from build123d import *

# Parameters (mm, degrees)
SKETCH_1_R          = 1.35
EXTRUDE_1_DEPTH     = 12.5
SKETCH_3_R          = 9
SKETCH_4_R          = 9.9
SKETCH_4_R_2        = 9
EXTRUDE_2_DEPTH     = 1
CUT_EXTRUDE_START   = -2
SKETCH_5_R          = 13.5
SKETCH_5_R_2        = 9.9
CUT_EXTRUDE_1_DEPTH = 2
SKETCH_6_R          = 10.1
CUT_EXTRUDE_2_DEPTH = 3.25
SKETCH_10_R         = 1.35
CUT_EXTRUDE_3_DEPTH = 8
CUT_EXTRUDE_4_REACH = 60.397
SKETCH_11_R         = 1.6
SKETCH_12_R         = 3
CUT_EXTRUDE_5_DEPTH = 4


with BuildPart() as part:
    # 草图1 → 凸台-拉伸1 (new, symmetric)
    with BuildSketch(Plane.XY):
        Polygon((0, 0), (0, 39.5), (-19, 39.5), (-35, 23.5), (-35, -20), (-17, -38), (0, -38), align=None)
        with Locations((-27.980762114, -15)):
            Circle(SKETCH_1_R, mode=Mode.SUBTRACT)
        with Locations((-23.213203436, -21.213203436)):
            Circle(SKETCH_1_R, mode=Mode.SUBTRACT)
        with Locations((-17, -25.980762114)):
            Circle(SKETCH_1_R, mode=Mode.SUBTRACT)
        with Locations((-9.764571353, -28.977774789)):
            Circle(SKETCH_1_R, mode=Mode.SUBTRACT)
        with Locations((-30.070163865, 15.944644586)):
            Circle(SKETCH_1_R, mode=Mode.SUBTRACT)
        with Locations((-26.212865417, 23.354445963)):
            Circle(SKETCH_1_R, mode=Mode.SUBTRACT)
        with Locations((-20.56920351, 29.51342218)):
            Circle(SKETCH_1_R, mode=Mode.SUBTRACT)
    extrude(amount=EXTRUDE_1_DEPTH, both=True)

    # 切除-扫描1: sweep along a path in 草图2
    with BuildLine(Plane.XY) as sweep_1_path:
        Line((0, -18), (-2, -18))
        ThreePointArc((-2, -18), (-14.727922061, -12.727922061), (-20, 0))
        Line((-20, 0), (-20, 5))
        ThreePointArc((-20, 5), (-17.320508076, 15), (-10, 22.320508076))
        ThreePointArc((-10, 22.320508076), (3.381115126, 27.650519119), (17.726426944, 28.94484851))
    # 草图3 → 切除-扫描1 (sweep, cut)
    with BuildSketch(Plane(origin=(0, 0, 0), x_dir=(0, 0, -1), z_dir=(1, 0, 0))):
        with Locations((0, -18)):
            Circle(SKETCH_3_R)
    sweep(path=sweep_1_path.line, mode=Mode.SUBTRACT)

    # 草图4 → 凸台-拉伸2 (add)
    with BuildSketch(Plane(origin=(0, 0, 0), x_dir=(0, 0, -1), z_dir=(1, 0, 0))):
        with Locations(Location((0, -18, 0), (0, 0, 180))):
            Circle(SKETCH_4_R)
        with Locations((0, -18)):
            Circle(SKETCH_4_R_2, mode=Mode.SUBTRACT)
    extrude(amount=EXTRUDE_2_DEPTH)

    # 草图5 → 切除-拉伸1 (cut)
    with BuildSketch(Plane(origin=(0, 0, 0), x_dir=(0, 0, -1), z_dir=(1, 0, 0)).offset(CUT_EXTRUDE_START)):
        with Locations((0, -18)):
            Circle(SKETCH_5_R)
        with Locations((0, -18)):
            Circle(SKETCH_5_R_2, mode=Mode.SUBTRACT)
    extrude(amount=CUT_EXTRUDE_1_DEPTH, mode=Mode.SUBTRACT)

    # 切除-扫描4: sweep along a path in 草图7
    with BuildLine(Plane.XY) as sweep_4_path:
        ThreePointArc((17.726426944, 28.94484851), (3.381115126, 27.650519119), (-10, 22.320508076))
    # 草图6 → 切除-扫描4 (sweep, cut)
    with BuildSketch(Plane(origin=(2.165063509, 1.25, 0), x_dir=(0, 0, -1), z_dir=(0.8660254037844397, 0.4999999999999983, 0))):
        with Locations((0, 24.330127019)):
            Circle(SKETCH_6_R)
    sweep(path=sweep_4_path.line, mode=Mode.SUBTRACT)

    # 草图9 → 切除-拉伸2 (cut, symmetric)
    with BuildSketch(Plane.XY):
        with BuildLine():
            ThreePointArc((-22.812131801, 25.903467515), (-17.697945128, 32.646850861), (-23.969937126, 26.964400628))
            ThreePointArc((-23.969937126, 26.964400628), (-29.694261605, 25.792145818), (-28.837986521, 20.012105587))
            ThreePointArc((-28.837986521, 20.012105587), (-32.032595471, 12.174848545), (-27.445042761, 19.286984962))
            ThreePointArc((-27.445042761, 19.286984962), (-22.731469229, 20.916746109), (-22.812131801, 25.903467515))
        make_face()
        with BuildLine():
            ThreePointArc((-24.286358775, -17.100924552), (-30.567998187, -11.628248304), (-26.907606774, -19.112278884))
            ThreePointArc((-26.907606774, -19.112278884), (-26.218407256, -24.218407256), (-21.112278884, -24.907606774))
            ThreePointArc((-21.112278884, -24.907606774), (-19.125, -29.66137008), (-14.014480772, -29.005522425))
            ThreePointArc((-14.014480772, -29.005522425), (-5.83808334, -30.604179376), (-12.750090581, -25.953014478))
            ThreePointArc((-12.750090581, -25.953014478), (-14.875, -22.300154147), (-19.100924552, -22.286358775))
            ThreePointArc((-19.100924552, -22.286358775), (-20.207999616, -18.207999616), (-24.286358775, -17.100924552))
        make_face()
    extrude(amount=CUT_EXTRUDE_2_DEPTH, both=True, mode=Mode.SUBTRACT)

    # 草图10 → 切除-拉伸3 (cut)
    with BuildSketch(Plane(origin=(0, 0, 0), x_dir=(0, 0, -1), z_dir=(1, 0, 0))):
        with Locations((-9, 7)):
            Circle(SKETCH_10_R)
        with Locations((9, 7)):
            Circle(SKETCH_10_R)
    extrude(amount=-CUT_EXTRUDE_3_DEPTH, mode=Mode.SUBTRACT)

    # 草图11 → 切除-拉伸4 (cut, up to next)
    with BuildSketch(Plane.XY.offset(12.5), mode=Mode.PRIVATE) as cut_extrude_4_sk1:
        with Locations((-20.56920351, 29.51342218)):
            Circle(SKETCH_11_R)
    cut_extrude_4_tool1 = extrude(cut_extrude_4_sk1.sketch, amount=-CUT_EXTRUDE_4_REACH, mode=Mode.PRIVATE) & part.part
    # 草图11 → 切除-拉伸4 (cut, up to next)
    with BuildSketch(Plane.XY.offset(12.5), mode=Mode.PRIVATE) as cut_extrude_4_sk2:
        with Locations((-26.212865417, 23.354445963)):
            Circle(SKETCH_11_R)
    cut_extrude_4_tool2 = extrude(cut_extrude_4_sk2.sketch, amount=-CUT_EXTRUDE_4_REACH, mode=Mode.PRIVATE) & part.part
    # 草图11 → 切除-拉伸4 (cut, up to next)
    with BuildSketch(Plane.XY.offset(12.5), mode=Mode.PRIVATE) as cut_extrude_4_sk3:
        with Locations((-30.070163865, 15.944644586)):
            Circle(SKETCH_11_R)
    cut_extrude_4_tool3 = extrude(cut_extrude_4_sk3.sketch, amount=-CUT_EXTRUDE_4_REACH, mode=Mode.PRIVATE) & part.part
    # 草图11 → 切除-拉伸4 (cut, up to next)
    with BuildSketch(Plane.XY.offset(12.5), mode=Mode.PRIVATE) as cut_extrude_4_sk4:
        with Locations((-27.980762114, -15)):
            Circle(SKETCH_11_R)
    cut_extrude_4_tool4 = extrude(cut_extrude_4_sk4.sketch, amount=-CUT_EXTRUDE_4_REACH, mode=Mode.PRIVATE) & part.part
    # 草图11 → 切除-拉伸4 (cut, up to next)
    with BuildSketch(Plane.XY.offset(12.5), mode=Mode.PRIVATE) as cut_extrude_4_sk5:
        with Locations((-23.213203436, -21.213203436)):
            Circle(SKETCH_11_R)
    cut_extrude_4_tool5 = extrude(cut_extrude_4_sk5.sketch, amount=-CUT_EXTRUDE_4_REACH, mode=Mode.PRIVATE) & part.part
    # 草图11 → 切除-拉伸4 (cut, up to next)
    with BuildSketch(Plane.XY.offset(12.5), mode=Mode.PRIVATE) as cut_extrude_4_sk6:
        with Locations((-17, -25.980762114)):
            Circle(SKETCH_11_R)
    cut_extrude_4_tool6 = extrude(cut_extrude_4_sk6.sketch, amount=-CUT_EXTRUDE_4_REACH, mode=Mode.PRIVATE) & part.part
    # 草图11 → 切除-拉伸4 (cut, up to next)
    with BuildSketch(Plane.XY.offset(12.5), mode=Mode.PRIVATE) as cut_extrude_4_sk7:
        with Locations((-9.764571353, -28.977774789)):
            Circle(SKETCH_11_R)
    cut_extrude_4_tool7 = extrude(cut_extrude_4_sk7.sketch, amount=-CUT_EXTRUDE_4_REACH, mode=Mode.PRIVATE) & part.part
    add(cut_extrude_4_tool1.solids().sort_by_distance((-20.569204, 29.513422, 12.5))[0], mode=Mode.SUBTRACT)
    add(cut_extrude_4_tool2.solids().sort_by_distance((-26.212865, 23.354446, 12.5))[0], mode=Mode.SUBTRACT)
    add(cut_extrude_4_tool3.solids().sort_by_distance((-30.070164, 15.944645, 12.5))[0], mode=Mode.SUBTRACT)
    add(cut_extrude_4_tool4.solids().sort_by_distance((-27.980762, -15, 12.5))[0], mode=Mode.SUBTRACT)
    add(cut_extrude_4_tool5.solids().sort_by_distance((-23.213203, -21.213203, 12.5))[0], mode=Mode.SUBTRACT)
    add(cut_extrude_4_tool6.solids().sort_by_distance((-17, -25.980762, 12.5))[0], mode=Mode.SUBTRACT)
    add(cut_extrude_4_tool7.solids().sort_by_distance((-9.764571, -28.977775, 12.5))[0], mode=Mode.SUBTRACT)

    # 草图12 → 切除-拉伸5 (cut)
    with BuildSketch(Plane.XY.offset(12.5)):
        with Locations((-20.56920351, 29.51342218)):
            Circle(SKETCH_12_R)
        with Locations((-26.212865417, 23.354445963)):
            Circle(SKETCH_12_R)
        with Locations((-30.070163865, 15.944644586)):
            Circle(SKETCH_12_R)
        with Locations((-27.980762114, -15)):
            Circle(SKETCH_12_R)
        with Locations((-23.213203436, -21.213203436)):
            Circle(SKETCH_12_R)
        with Locations((-17, -25.980762114)):
            Circle(SKETCH_12_R)
        with Locations((-9.764571353, -28.977774789)):
            Circle(SKETCH_12_R)
    extrude(amount=-CUT_EXTRUDE_5_DEPTH, mode=Mode.SUBTRACT)


solid = part.part
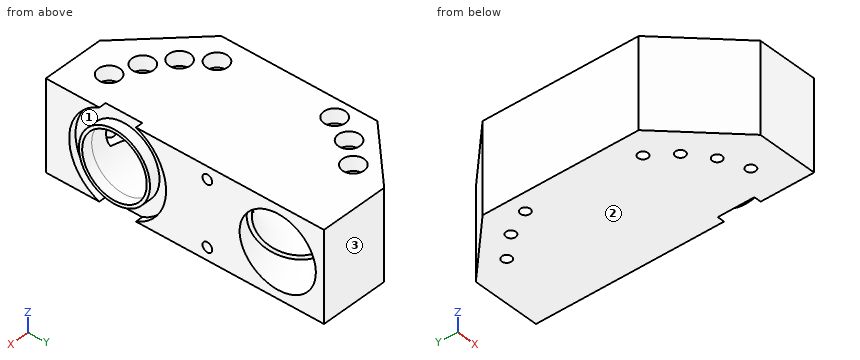
Input: part model. Units: mm. Frame: model coordinates. Face numbers are marked on the shaded views. Round coordinates to 2 decimals unless told otherwise and drop trailing zeros.
1. Pin query (flat end, axial travel): P1, Ø1.8, axis at x = -30.5, y = 15.5, coming from the +Z side; P2, Ø5, axis at x = -20.57, y = 29.51, coming from the +Z side; P3, Ø2, axis at x = -26.21, y = 23.35, coming from the -Z side; P4, Ø3, axis at y = 24.5, z = -0.5, coming from the +X side. Return the tip coordinate at first contact, or that it passes through.
The answers:
P1: stops at z = -3.25
P2: stops at z = 8.5
P3: passes through
P4: stops at x = -20.49
2. Mould query, pull axis Z, two halves, no side actions, for the marked faces 1, 2 and 3. Classes: released by +Z, released by -Z, zero draft, split by the parting line, or undercut.
The answers:
face 1: undercut
face 2: released by -Z
face 3: zero draft
3. Material intervals for line 1 (Z direction, x = -8.5, y = 25.5); line 2 (Y direction, x = -17, z = 6.25); line 3 (X direction, y = -27.5, z = -1.5), sorted ascending.
The answers:
line 1: z = -12.5 to -9.88, 9.88 to 12.5
line 2: y = -38 to -27.58, -24.38 to -19.34, 25.3 to 39.5
line 3: x = -27.5 to -20.97, -5.78 to 1
